Check sheet for the modelled part. Datum: model origin and axes. Units: mm. Coordinates: 2 decimals unless noted, no trailing zeros. Order: outer loops, then holes, each group sorted by start corner. A loop starts at its lowest first (then second) coordinate and runs counter-clockwise, first axis right, second up.
from build123d import *

# Parameters (mm, degrees)
SKICA1_R                 = 0.5
SKICA1_R_2               = 2.3
SKICA1_R_3               = 0.9
SKICA1_W                 = 3
SKICA1_H                 = 13
SKICA1_H_2               = 5.5
SKICA1_W_2               = 17.6
SKICA1_H_3               = 10.6
SKICA1_W_3               = 12.4
SKICA1_H_4               = 24
SKICA1_W_4               = 2.8
SKICA1_W_5               = 3.2
SKICA1_H_5               = 10
SKICA1_W_6               = 4.6
SKICA1_H_6               = 4.6
P_IDAT_VYSUNUT_M1_DEPTH  = 3
SKICA2_R                 = 1.5
ODEBRAT_VYSUNUT_M1_DEPTH = 3
ZKOSEN_1_SIZE            = 1.5
ZAOBLIT1_R               = 40
ZAOBLIT2_R               = 4
SKICA3_R                 = 0.5
SKICA3_W                 = 2.8
SKICA3_H                 = 13
ODEBRAT_VYSUNUT_M2_DEPTH = 129.730338305


with BuildPart() as part:
    # Skica1 → Přidat vysunutím1 (new body)
    with BuildSketch(Plane.XY):
        Polygon((-62.5, -32.5), (-62.5, 32.5), (-32.5, 62.5), (-19.003438856, 112.5), (19.003438856, 112.5), (32.5, 62.5), (62.5, 32.5), (62.5, -32.5), (32.5, -62.5), (-32.5, -62.5), align=None)
        with Locations((0, 100.5)):
            Circle(SKICA1_R, mode=Mode.SUBTRACT)
        with Locations(Location((0, 72.5, 0), (0, 0, 180))):
            Circle(SKICA1_R, mode=Mode.SUBTRACT)
        with Locations((0, 108.5)):
            Circle(SKICA1_R_2, mode=Mode.SUBTRACT)
        with Locations((7.97, 108.5)):
            Circle(SKICA1_R_2, mode=Mode.SUBTRACT)
        with Locations((15.94, 108.5)):
            Circle(SKICA1_R_2, mode=Mode.SUBTRACT)
        with Locations(Location((-15.94, 108.5, 0), (0, 0, 180))):
            Circle(SKICA1_R_2, mode=Mode.SUBTRACT)
        with Locations(Location((-7.97, 108.5, 0), (0, 0, 180))):
            Circle(SKICA1_R_2, mode=Mode.SUBTRACT)
        with Locations(Location((-18.017013584, 100.805397049, 0), (0, 0, 180))):
            Circle(SKICA1_R_2, mode=Mode.SUBTRACT)
        with Locations((-20.094027168, 93.110794098)):
            Circle(SKICA1_R_2, mode=Mode.SUBTRACT)
        with Locations((-22.171040752, 85.416191147)):
            Circle(SKICA1_R_2, mode=Mode.SUBTRACT)
        with Locations((-24.248054336, 77.721588196)):
            Circle(SKICA1_R_2, mode=Mode.SUBTRACT)
        with Locations(Location((24.248054336, 77.721588196, 0), (0, 0, 180))):
            Circle(SKICA1_R_2, mode=Mode.SUBTRACT)
        with Locations(Location((22.171040752, 85.416191147, 0), (0, 0, 180))):
            Circle(SKICA1_R_2, mode=Mode.SUBTRACT)
        with Locations(Location((20.094027168, 93.110794098, 0), (0, 0, 180))):
            Circle(SKICA1_R_2, mode=Mode.SUBTRACT)
        with Locations((18.017013584, 100.805397049)):
            Circle(SKICA1_R_2, mode=Mode.SUBTRACT)
        with Locations((47.397781356, 0)):
            Circle(SKICA1_R_3, mode=Mode.SUBTRACT)
        with Locations(Location((26.897781356, 0, 0), (0, 0, 180))):
            Circle(SKICA1_R_3, mode=Mode.SUBTRACT)
        with Locations(Location((-47.397781356, 0, 0), (0, 0, 180))):
            Circle(SKICA1_R_3, mode=Mode.SUBTRACT)
        with Locations((-26.897781356, 0)):
            Circle(SKICA1_R_3, mode=Mode.SUBTRACT)
        Polygon((-44.147781356, 3.2), (-38.647781356, 3.2), (-38.647781356, 7.5), (-35.647781356, 7.5), (-35.647781356, 3.2), (-30.147781356, 3.2), (-30.147781356, -3.2), (-35.647781356, -3.2), (-35.647781356, -7.5), (-38.647781356, -7.5), (-38.647781356, -3.2), (-44.147781356, -3.2), align=None, mode=Mode.SUBTRACT)
        with Locations((-43.047781356, 20.7)):
            Rectangle(SKICA1_W, SKICA1_H, mode=Mode.SUBTRACT)
        with Locations((-52.847781356, 0)):
            Rectangle(SKICA1_W, SKICA1_H_2, mode=Mode.SUBTRACT)
        with Locations((-43.047781356, -20.7)):
            Rectangle(SKICA1_W, SKICA1_H, mode=Mode.SUBTRACT)
        Polygon((38.647781356, -7.5), (35.647781356, -7.5), (35.647781356, -3.2), (30.147781356, -3.2), (30.147781356, 3.2), (35.647781356, 3.2), (35.647781356, 7.5), (38.647781356, 7.5), (38.647781356, 3.2), (44.147781356, 3.2), (44.147781356, -3.2), (38.647781356, -3.2), align=None, mode=Mode.SUBTRACT)
        with Locations((52.847781356, 0)):
            Rectangle(SKICA1_W, SKICA1_H_2, mode=Mode.SUBTRACT)
        with Locations((43.047781356, 20.7)):
            Rectangle(SKICA1_W, SKICA1_H, mode=Mode.SUBTRACT)
        with Locations((43.047781356, -20.7)):
            Rectangle(SKICA1_W, SKICA1_H, mode=Mode.SUBTRACT)
        with Locations((16.7, 53.8)):
            Rectangle(SKICA1_W_2, SKICA1_H_3, mode=Mode.SUBTRACT)
        with Locations((0, 28.8)):
            Rectangle(SKICA1_W_2, SKICA1_H_3, mode=Mode.SUBTRACT)
        with Locations((-16.7, 53.8)):
            Rectangle(SKICA1_W_2, SKICA1_H_3, mode=Mode.SUBTRACT)
        with Locations((0, 86.5)):
            Rectangle(SKICA1_W_3, SKICA1_H_4, mode=Mode.SUBTRACT)
        with Locations((-12.4, 86.5)):
            Rectangle(SKICA1_W_4, SKICA1_H, mode=Mode.SUBTRACT)
        Polygon((-20.487479207, 65.088190451), (-10.828220944, 62.5), (-10, 65.590962644), (-19.659258263, 68.179153095), align=None, mode=Mode.SUBTRACT)
        with Locations((12.4, 86.5)):
            Rectangle(SKICA1_W_4, SKICA1_H, mode=Mode.SUBTRACT)
        with Locations((31.6, 31)):
            Rectangle(SKICA1_W_5, SKICA1_H_5, mode=Mode.SUBTRACT)
        with Locations((-31.6, 31)):
            Rectangle(SKICA1_W_5, SKICA1_H_5, mode=Mode.SUBTRACT)
        with Locations((25.3, 20.23)):
            Rectangle(SKICA1_W_6, SKICA1_H_6, mode=Mode.SUBTRACT)
        with Locations((25.3, -51.5)):
            Rectangle(SKICA1_W_6, SKICA1_H_6, mode=Mode.SUBTRACT)
        with Locations((-25.3, -51.5)):
            Rectangle(SKICA1_W_6, SKICA1_H_6, mode=Mode.SUBTRACT)
        with Locations((-25.3, 20.23)):
            Rectangle(SKICA1_W_6, SKICA1_H_6, mode=Mode.SUBTRACT)
    extrude(amount=P_IDAT_VYSUNUT_M1_DEPTH)

    # Skica2 → Odebrat vysunutím1 (cut)
    with BuildSketch(Plane.XY):
        with Locations(Location((0, 39.6, 0), (0, 0, 180))):
            Circle(SKICA2_R)
        with Locations(Location((0, 55.6, 0), (0, 0, 180))):
            Circle(SKICA2_R)
        with Locations(Location((0, -55.6, 0), (0, 0, 180))):
            Circle(SKICA2_R)
        with Locations(Location((0, -39.6, 0), (0, 0, 180))):
            Circle(SKICA2_R)
    extrude(amount=ODEBRAT_VYSUNUT_M1_DEPTH, mode=Mode.SUBTRACT)

    # Zkosení1
    zkosen_1_edges = [part.edges().sort_by_distance(p)[0] for p in [
        (1.5, 55.6, 3),
        (1.5, -55.6, 3),
        (1.5, -39.6, 3),
        (1.5, 39.6, 3),
    ]]
    chamfer(zkosen_1_edges, length=ZKOSEN_1_SIZE)

    # Zaoblit1
    zaoblit1_edges = [part.edges().sort_by_distance(p)[0] for p in [
        (-62.5, -32.5, 1.5),
        (-62.5, 32.5, 1.5),
        (-32.5, 62.5, 1.5),
        (32.5, 62.5, 1.5),
        (62.5, 32.5, 1.5),
        (62.5, -32.5, 1.5),
        (32.5, -62.5, 1.5),
        (-32.5, -62.5, 1.5),
    ]]
    fillet(zaoblit1_edges, radius=ZAOBLIT1_R)

    # Zaoblit2
    zaoblit2_edges = [part.edges().sort_by_distance(p)[0] for p in [
        (-19.003438856, 112.5, 1.5),
        (19.003438856, 112.5, 1.5),
    ]]
    fillet(zaoblit2_edges, radius=ZAOBLIT2_R)

    # Skica3 → Odebrat vysunutím2 (cut, through all)
    with BuildSketch(Plane.XY.offset(3)):
        with Locations((-28.2, 41.3)):
            Circle(SKICA3_R)
        with Locations(Location((28.2, 41.3, 0), (0, 0, 180))):
            Circle(SKICA3_R)
        with Locations((0, -50.6)):
            Rectangle(SKICA3_W, SKICA3_H)
    extrude(amount=-ODEBRAT_VYSUNUT_M2_DEPTH, mode=Mode.SUBTRACT)


solid = part.part
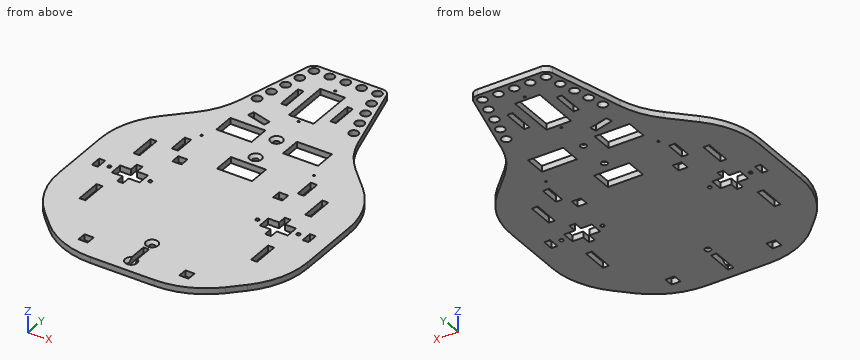
(1) Go/stop test with flat-tipped pins: P1, Ø1.5, axis at y = 19, z = 2, coming from the -X side; P2, Ø5, axis at x = -26.5, y = -24.5, coming from the -Z side; P3, Ø2.5, axis at x = 0, y = 39.6, coming from the +Z side; P4, Ø1.5, axis at y = 94, z = 2.5, coming from the -X side. Record where each tip stops, or that it passes through.
Filled in:
P1: stops at x = -62.43
P2: stops at z = 0
P3: passes through
P4: stops at x = -24.2
(2) Cross-section at A-A (y = -29.5). Enter the section's corners in (x, z), and give its area (3 significant figures).
Filled in:
outline: (-60.13, 0) - (60.13, 0) - (60.13, 3) - (-60.13, 3) - close
area: 361 mm2
(3) Thickness scan on probe 1 along Y at (x, z) = (5, 1.1); probe 2 along Y at (x, z) = (15.94, 0.6); probe 3 along Y at (x, z) = (-14.5, 2.35). Record the ranges inside material, lowest first.
Filled in:
probe 1: y = -62.5 to 23.5, 34.1 to 74.5, 98.5 to 112.5
probe 2: y = -62.5 to 48.5, 59.1 to 99.82, 101.79 to 106.2, 110.8 to 112.5
probe 3: y = -62.5 to 48.5, 59.1 to 63.48, 66.8 to 106.71, 110.29 to 112.5
